```python
from build123d import *

# Parameters (mm, degrees)
BOSS_EXTRUDE1_DEPTH = 4
SKETCH2_R           = 1.625
CUT_EXTRUDE1_DEPTH  = 51.159744816


with BuildPart() as part:
    # Sketch1 → Boss-Extrude1 (new body)
    with BuildSketch(Plane.XY):
        with BuildLine():
            Line((0, 35), (0, 40))
            Line((0, 40), (-15, 40))
            ThreePointArc((-15, 40), (-25.606601718, 35.606601718), (-30, 25))
            Line((-30, 25), (-30, 0))
            Line((-30, 0), (0, 0))
            Line((0, 0), (0, 35))
        make_face()
    extrude(amount=BOSS_EXTRUDE1_DEPTH)

    # Sketch2 → Cut-Extrude1 (cut, through all)
    with BuildSketch(Plane.XY.offset(4)):
        with Locations((-7, 23)):
            Circle(SKETCH2_R)
        with Locations((-7, 13)):
            Circle(SKETCH2_R)
    extrude(amount=-CUT_EXTRUDE1_DEPTH, mode=Mode.SUBTRACT)


solid = part.part
```
Here's how the part is built. I have some questions about the finished solid (model axes, mm). Coordinates: 2 decimals unless noted, no trailing zeros. Write each loop counter-clockwise with the first axis right and the second up, starting at its lowest first coordinate (ties: lowest second). Pieces come first, ordered by that corner, then holes. Notation, with made-up numbers: (64, 73.5) -> (93, 73.5) arc R21 ccw to (93, 80.5) -> close; hole circle Ø10 at (-29, 70). An arc over 180 degrees is marked (long way). Use a Markdown table: item, result. Add a question column.
(1) If we section it at A-A, the plane y = 13: Write out the boundary of the cut face in (x, z) (3 decimals).
(2) If we section it at B-B, the plane x = -7: Write out the boundary of the cut face in (y, z) (3 decimals).
(3) We'd pull the mould along X, two halves only. Please class faces 1 (the cylindrical face through (-7.352, 11.414, 2.028)), 2 (the flat face through (-30, 13, 2)), 3 (the flat face through (-15, 20, 0)), 4 (the cylindrical face through (-7.352, 21.414, 2.028)): +X half, -X half, draft (parallel to the pull), parting line (faces both ways), or undercut.
(4) If we section it at D-D, the plane y = 34: Write out the boundary of the cut face in (x, z), and give its area (3 significant figures).
(5) I'm going to push a flat-ended pin straight in: P1, Ø1, axis at y = 30.5, z = 2.5, coming from the +X side. Where does the tip first touch, or does it pass through?
(6) If we section it at C-C, the plane z = 2.55: Write out the boundary of the cut face in (x, y) (3 decimals).
(7) Please list where these lines run through material, in increasing order: line 1 (Y direction, x = -7, z = 3.1) (3 decimals); line 2 (X direction, y = 25.5, z = 0.45); line 3 (Y direction, x = -23.75, z = 1.3).
Outcome:
| question | item | result |
|---|---|---|
| 1 | outline | (-30, 0) -> (-8.625, 0) -> (-8.625, 4) -> (-30, 4) -> close; (-5.375, 0) -> (0, 0) -> (0, 4) -> (-5.375, 4) -> close |
| 2 | outline | (0, 0) -> (11.375, 0) -> (11.375, 4) -> (0, 4) -> close; (14.625, 0) -> (21.375, 0) -> (21.375, 4) -> (14.625, 4) -> close; (24.625, 0) -> (40, 0) -> (40, 4) -> (24.625, 4) -> close |
| 3 | face 1 | undercut |
| 3 | face 2 | -X half |
| 3 | face 3 | draft |
| 3 | face 4 | undercut |
| 4 | outline | (-27, 0) -> (0, 0) -> (0, 4) -> (-27, 4) -> close |
| 4 | area | 108 mm^2 |
| 5 | P1 | stops at x = 0 |
| 6 | outline | (-30, 0) -> (0, 0) -> (0, 40) -> (-15, 40) arc R15 ccw to (-30, 25) -> close; hole circle Ø3.25 at (-7, 13); hole circle Ø3.25 at (-7, 23) |
| 7 | line 1 | y = 0 to 11.375, 14.625 to 21.375, 24.625 to 40 |
| 7 | line 2 | x = -29.99 to 0 |
| 7 | line 3 | y = 0 to 37.18 |
